Autodesk Inventor part; units mm, degrees
ref_plane "YZ Plane" through (0, 0, 0) normal (1, 0, 0) x (0, 1, 0)
ref_plane "XZ Plane" through (0, 0, 0) normal (0, 1, 0) x (-1, 0, 0)
ref_plane "XY Plane" through (0, 0, 0) normal (0, 0, 1) x (1, 0, 0)
sketch "Sketch1" plane through (0, 0, 0) normal (0, 0, 1) x (1, 0, 0)
  line L0 (-11.1895, 18.0847) -> (3.8105, 18.0847)
  line L1 (3.8105, 18.0847) -> (3.8105, -41.9153)
  line L2 (3.8105, -41.9153) -> (-11.1895, -41.9153)
  line L3 (-11.1895, -41.9153) -> (-11.1895, 18.0847)
  point P0 (0, 0)
  dimension "d0" = 15
  dimension "d1" = 60
extrude "Extrusion1" add sketch "Sketch1" along normal blind 2
sketch "Sketch2" plane through (-11.1895, -41.9153, 0) normal (0, -1, 0) x (1, 0, 0)
  line L0 (0, 2) -> (15, 2)
  line L1 (0, 2) -> (15, 2)
  line L2 (15, 2) -> (15, -4)
  line L3 (15, -4) -> (0, -4)
  line L4 (0, -4) -> (0, 2)
  line L5 (15, 0) -> (15, 2)
  point P0 (11.1895, 0)
  dimension "d4" = 6
extrude "Extrusion2" add sketch "Sketch2" against normal blind 3
sketch "Sketch3" plane through (-11.1895, 18.0847, 0) normal (0, 1, 0) x (1, 0, 0)
  line L0 (0, -2) -> (15, -2)
  line L1 (0, -2) -> (0, 4)
  line L2 (15, -2) -> (0, -2)
  line L3 (0, -2) -> (0, 4)
  line L4 (0, 4) -> (15, 4)
  line L5 (15, 4) -> (15, -2)
  point P0 (11.1895, 0)
extrude "Extrusion3" add sketch "Sketch3" against normal blind 3
chamfer "Chamfer1" distance 3 angle 45 2 edges at (-3.6895, 15.0847, 0) (-3.6895, -38.9153, 0)
sketch "Sketch4" plane through (-11.1895, -41.9153, 2) normal (0, -1, 0) x (1, 0, 0)
  line L0 (15, -6) -> (15, 0)
  line L1 (0, 0) -> (15, 0)
  point P0 (11.1895, -2)
  point P1 (12, -3)
  point P2 (3, -3)
  dimension "d12" = 3
  dimension "d13" = 12
  dimension "d14" = 3
  dimension "d15" = 3
hole "Hole1" at (0.8105, -41.9153, -1) at (-8.1895, -41.9153, -1) direction (0, 1, 0) diameter 2 depth 3 tip angle 118
sketch "Sketch5" plane through (-11.1895, 18.0847, 2) normal (0, 1, 0) x (1, 0, 0)
  circle A0 centre (12, 3) radius 1
  circle A1 centre (3, 3) radius 1
  point P0 (11.1895, 2)
hole "Hole2" at (0.8105, 18.0847, -1) at (-8.1895, 18.0847, -1) direction (0, -1, 0) diameter 2 depth 3 tip angle 118
sketch "Sketch6" plane through (0, 0, 2) normal (0, 0, 1) x (1, 0, 0)
  line L0 (3.8105, -41.9153) -> (-11.1895, -41.9153)
  line L1 (-11.1895, -41.9153) -> (-11.1895, -41.8153)
  line L2 (-11.1895, -41.8153) -> (3.8105, -41.8153)
  line L3 (3.8105, -41.8153) -> (3.8105, -41.9153)
  line L4 (3.8105, 17.9847) -> (-11.1895, 17.9847)
  line L5 (-11.1895, 17.9847) -> (-11.1895, 18.0847)
  line L6 (-11.1895, 18.0847) -> (3.8105, 18.0847)
  line L7 (3.8105, 18.0847) -> (3.8105, 17.9847)
  line L8 (3.8105, -41.9153) -> (3.8105, 18.0847)
  line L9 (3.8105, 18.0847) -> (-11.1895, 18.0847)
  line L10 (-11.1895, 18.0847) -> (-11.1895, -41.9153)
  line L11 (-11.1895, -41.9153) -> (3.8105, -41.9153)
  point P0 (0, 0)
  dimension "d30" = 0.1
  dimension "d31" = 0.1
extrude "Extrusion4" cut sketch "Sketch6" against normal blind 30 contours L0 L1 L2 L3 | L4 L5 L6 L7
chamfer "Chamfer2" distance 2 angle 45 2 edges at (3.8105, -40.3653, -4) (3.8105, 16.5347, -4)
chamfer "Chamfer3" distance 2 angle 45 2 edges at (-11.1895, 16.5347, -4) (-11.1895, -40.3653, -4)
sketch "Sketch7" plane through (0, 0, 2) normal (0, 0, 1) x (1, 0, 0)
  line L0 (3.8105, -41.8153) -> (3.8105, 17.9847)
  line L1 (3.8105, -2.0153) -> (0.8105, -2.0153)
  line L2 (0.8105, -2.0153) -> (0.8105, -21.8153)
  line L3 (0.8105, -21.8153) -> (3.8105, -21.8153)
  line L4 (3.8105, -21.8153) -> (3.8105, -2.0153)
  line L5 (3.8105, 17.9847) -> (-11.1895, 17.9847)
  line L6 (-11.1895, -41.8153) -> (3.8105, -41.8153)
  point P0 (0, 0)
  dimension "d40" = 3
  dimension "d41" = 20
  dimension "d42" = 20
extrude "Extrusion5" cut sketch "Sketch7" against normal blind 2
chamfer "Chamfer4" distance 3 angle 45 2 edges at (3.8105, -2.0153, 1) (3.8105, -21.8153, 1)
sketch "Sketch8" plane through (0, 0, 2) normal (0, 0, 1) x (1, 0, 0)
  line L0 (-11.1895, 14.0847) -> (-11.1895, 17.9847)
  line L1 (-11.1895, 17.9847) -> (-21.1895, 17.9847)
  line L2 (-21.1895, 17.9847) -> (-21.1895, -41.8153)
  line L3 (-21.1895, -41.8153) -> (-11.1895, -41.8153)
  line L4 (-11.1895, -41.8153) -> (-11.1895, 17.9847)
  line L5 (-11.1895, -41.8153) -> (3.8105, -41.8153)
  point P0 (0, 0)
  dimension "d48" = 10
extrude "Extrusion6" add sketch "Sketch8" against normal blind 1.2
chamfer "Chamfer5" distance 0.8 angle 45 1 edges at (-11.1895, -11.9153, 0)
sketch "Sketch9" plane through (0, 0, 0.8) normal (0, 0, -1) x (-1, 0, 0)
  line L0 (9.1895, 15.0847) -> (9.1895, 17.9847)
  line L1 (21.1895, 17.9847) -> (21.1895, -41.8153)
  line L2 (9.1895, 17.9847) -> (21.1895, 17.9847)
  line L3 (21.1895, 17.9847) -> (21.1895, 15.9847)
  line L4 (21.1895, 15.9847) -> (9.1895, 15.9847)
  line L5 (9.1895, 15.9847) -> (9.1895, 17.9847)
  line L6 (9.1895, -38.9153) -> (9.1895, -41.8153)
  line L7 (9.1895, -41.8153) -> (21.1895, -41.8153)
  line L8 (21.1895, -41.8153) -> (21.1895, -39.8153)
  line L9 (21.1895, -39.8153) -> (9.1895, -39.8153)
  line L10 (9.1895, -39.8153) -> (9.1895, -41.8153)
  line L11 (21.1895, 17.9847) -> (11.1895, 17.9847)
  point P0 (0, 0)
  point P1 (21.1895, -39.8153)
  point P2 (9.1895, -39.8153)
  point P3 (9.1895, 15.9847)
  dimension "d54" = 2
  dimension "d55" = 2
extrude "Extrusion7" add sketch "Sketch9" along normal blind 4.8
chamfer "Chamfer6" distance 2 angle 45 2 edges at (-21.1895, -40.8153, -4) (-21.1895, 16.9847, -4)
sketch "Sketch10" plane through (0, 0, 0.8) normal (0, 0, -1) x (-1, 0, 0)
  line L0 (11.1895, -39.8153) -> (11.1895, -35.1153)
  line L1 (11.1895, -37.8153) -> (19.1895, -37.8153)
  line L2 (19.1895, -37.8153) -> (19.1895, 13.9847)
  line L3 (19.1895, 13.9847) -> (11.1895, 13.9847)
  line L4 (11.1895, 13.9847) -> (11.1895, -37.8153)
  line L5 (9.1895, 15.9847) -> (19.1895, 15.9847)
  line L6 (21.1895, -39.8153) -> (21.1895, 15.9847)
  line L7 (19.1895, -39.8153) -> (9.1895, -39.8153)
  point P0 (0, 0)
  dimension "d61" = 2
  dimension "d62" = 2
  dimension "d63" = 2
extrude "Extrusion8" cut sketch "Sketch10" against normal blind 2
fillet "Fillet1" radius 2 2 edges at (-11.1895, 13.9847, 1.4) (-11.1895, -37.8153, 1.4)
sketch "Sketch12" plane through (0, 0, 2) normal (0, 0, 1) x (1, 0, 0)
  line L0 (-11.1895, -35.1153) -> (-11.1895, 11.2847)
  line L1 (-19.1895, 13.9847) -> (-13.1895, 13.9847)
  line L2 (-13.1895, -37.8153) -> (-19.1895, -37.8153)
  line L3 (-19.1895, -37.8153) -> (-19.1895, 13.9847)
  line L4 (-19.1895, -37.8153) -> (-10.1895, -11.9153) construction
  line L5 (-18.2449, -38.1436) -> (-9.2449, -12.2436)
  line L6 (-11.1341, -11.5871) -> (-20.1341, -37.4871)
  arc A0 (-20.1341, -37.4871) -> (-18.2449, -38.1436) centre (-19.1895, -37.8153) ccw
  arc A1 (-9.2449, -12.2436) -> (-11.1341, -11.5871) centre (-10.1895, -11.9153) ccw
  line L7 (-10.1895, -11.9153) -> (-19.1895, 13.9847) construction
  line L8 (-9.2449, -11.5871) -> (-18.2449, 14.3129)
  line L9 (-20.1341, 13.6564) -> (-11.1341, -12.2436)
  arc A2 (-11.1341, -12.2436) -> (-9.2449, -11.5871) centre (-10.1895, -11.9153) ccw
  arc A3 (-18.2449, 14.3129) -> (-20.1341, 13.6564) centre (-19.1895, 13.9847) ccw
  point P0 (0, 0)
  point P1 (-11.1895, -11.9153)
  point P2 (-14.6895, -24.8653)
  point P3 (-14.6895, 1.0347)
  point P4 (-19.1895, 10.9381)
  point P5 (-11.2482, -11.9153)
  point P6 (-19.1895, -34.7688)
  point P7 (-18.1309, -37.8153)
  point P8 (-11.1895, -17.8397)
  point P9 (-11.1895, -5.991)
  point P10 (-18.1309, 13.9847)
  dimension "d71" = 1
  dimension "d72" = 51.8
  dimension "d73" = 25.9
  dimension "d74" = 2
  dimension "d75" = 2
extrude "Extrusion10" add sketch "Sketch12" against normal blind 1.2 contours L5 L2 L3 L6 L9 L0 | L9 L6 L0 | L6 L9 L3 L1 L8 L0
properties part number "structural-bar"
Check sheet for the modelled part. Datum: model origin and axes. Units: mm. A direction names the side the tool comes from. Round coordinates to 2 decimals unless told otherwise and drop trailing zeros. Loops run counter-clockwise (first coordinate to the right, second up) from the corner with the lowest first, then second, coordinate; pieces in that order, holes last. Notation, with made-up numbers: (-21, -26) - (-5, -26) arc R24 cw to (-5, 6) - close; hole circle Ø1 at (8, 76.5). An arc over 180 degrees is marked (long way). Write item = value, one per line. Start each with the question number.
Q1. Section check C-C (x = -17.5). Record the boundary of the cut face in (y, z).
Q2. Release check for a two-part mould opening along X. For faces 6 (the face through (-21.19, -12, 1)), 7 (the face through (-15, -39.815, -2)), 8 (the face through (1.787, -40.345, -0.783)) record: pulls with the +X half, pulls with the -X half, needs draft (parallel to the pull), parting line crosses it, or undercut.
Q3. Section check A-A (x = -2). Record the boundary of the cut face in (y, z), plus the area to 3 significant figures.
Q4. Thickness scan on L1, parallel to X at y = 16.1, z = -1; L2, parallel to X at y = -39.6, z = -1; L3, parallel to Y at x = -12.5, z = -2.25. Record the ranges inside material, lowest first.
Q5. Depth check by flat-ended pin: P1, Ø2, axis at x = -0.5, y = -9, coming from the -Z side; P2, Ø1, axis at y = -9.5, z = 1, coming from the +X side; P3, Ø1.6, axis at x = 0.81, z = -1, coming from the +Y side; P4, Ø3, axis at y = 7, z = -2.5, coming from the -X side. Enter the tip coordinate at first touch or a pass-through.
Q6. Section check B-B (y = -21). Record the boundary of the cut face in (x, z) (1 decimal).
Q7. Access from +Z, -Z, +X, -X, +Y, -Y to the whole of each face (thin tool, end or side, straight path). Record for faces 1 (the face through (-11.791, -37.245, 1.408)), 2 (the face through (1.787, 16.514, -1.217)), 3 (the face through (2.332, -23.336, 1.014)), 4 (the face through (-15, 15.985, -2)), 5 (the face through (-3.8, 15.085, -3.5)).
Derived:
q1.outline = (-41.82, -4) - (-39.82, -4) - (-39.82, 0.8) - (-37.82, 0.8) - (-37.82, 2) - (-41.82, 2) - close; (-36, 0.8) - (-29.91, 0.8) - (-29.91, 2) - (-36, 2) - close; (6.08, 0.8) - (12.17, 0.8) - (12.17, 2) - (6.08, 2) - close; (13.98, 0.8) - (15.98, 0.8) - (15.98, -4) - (17.98, -4) - (17.98, 2) - (13.98, 2) - close
q2.face_6 = pulls with the -X half
q2.face_7 = needs draft
q2.face_8 = undercut
q3.outline = (-41.82, -4) - (-38.92, -4) - (-38.92, -3) - (-35.92, 0) - (12.08, 0) - (15.08, -3) - (15.08, -4) - (17.98, -4) - (17.98, 2) - (-41.82, 2) - close
q3.area = 152 mm^2
q4.L1 = -21.19 to -9.19, -7.19 to -0.19, 1.81 to 3.81
q4.L2 = -11.19 to -9.19, -7.19 to -0.19, 1.81 to 3.81
q4.L3 = -41.82 to -39.82, 15.98 to 17.98
q5.P1 = 0
q5.P2 = 0.81
q5.P3 = 14.96
q5.P4 = through
q6.outline = (-21.2, 0.8) - (-19.2, 0.8) - (-19.2, 2) - (-21.2, 2) - close; (-14.4, 0.8) - (-12.3, 0.8) - (-12.3, 2) - (-14.4, 2) - close; (-11.2, 0.8) - (-10.4, 0) - (0.8, 0) - (0.8, 2) - (-11.2, 2) - close
q7.face_1 = +Z, -Z
q7.face_2 = +Y
q7.face_3 = +Z, -Z, +X
q7.face_4 = -Z, -X
q7.face_5 = -Z, +X, -X
